Verification items for this drawing (mm, ordinates from the low corner). A direction names the side the tool comes from. Round coordinates to 2 decimals unless told otherwise and drop trailing zeros. Order: outer loops, then holes, each group sorted by start corner. A loop starts at its lowest first (then second) coordinate and runs counter-clockwise, first axis right, second up. Notation, with made-up numbers: (-13.75, 55) - (9.25, 55) arc R10 ccw to (9.25, 62) - close; hole circle Ø8 at (73.25, 43). An arc over 180 degrees is marked (long way). Return JSON: item names as keys, results as strings. Group by question number.
Q1. Sectioned sample at B-B, the plane y = 9. Record the cut outline in (x, z), then the cut area to 3 significant figures.
Q2. Sectioned sample at D-D, the plane x = 6. Record the cut outline in (y, z).
Q3. Draft check along X on the marked faces 4, 5 and 6. Enter one of: pulls with the +X half, pulls with the -X half, needs draft (parallel to the pull), parting line crosses it, or undercut.
Q4. Tool access check on the marked faces 1, 2 and 3. Record the directions out of +Z, -Z, +X, -X, +Y, -Y that give a thin tool (end or side, any length) a straight path to the whole face; none if there is none.
Q5. Gauge pin test, flat ends, axial feed: pin 1 Ø8 at (y, z) = (7.5, 35) entering from +X; pin 2 Ø3 at (x, y) = (58, 18) entering from -Z; pin 3 Ø1.5 at (x, z) = (1.5, 42.5) entering from -Y. Record the tip position at first contact, or that the pin passes through.
Q6. Sectioned sample at A-A, the plane z = 58.75. Record the cut outline in (x, y).
Q7. Material ranges on line 1 along Z through (x, y) = (5, 20); line 2 along X through (y, z) = (1.5, 66.5); line 3 along X through (y, z) = (15.5, 69.5), recorded low to high.
Q8. Sectioned sample at C-C, the plane y = 18.75. Record the cut outline in (x, z).
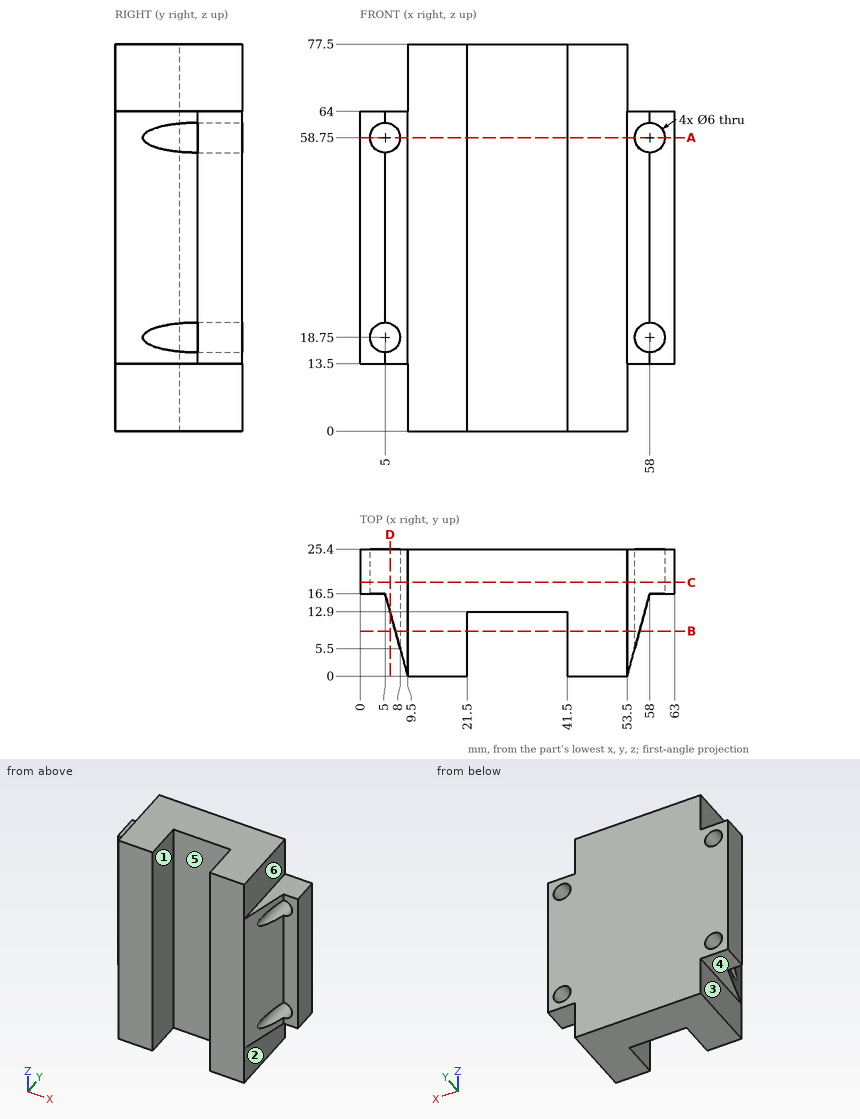
Reply:
{
 "1": {"outline": "(7.05, 13.5) - (9.5, 13.5) - (9.5, 0) - (21.5, 0) - (21.5, 77.5) - (9.5, 77.5) - (9.5, 64) - (7.05, 64) - (7.05, 60.94) arc R3 cw to (7.05, 56.56) - (7.05, 20.94) arc R3 cw to (7.05, 16.56) - close; (41.5, 0) - (53.5, 0) - (53.5, 13.5) - (55.95, 13.5) - (55.95, 16.56) arc R3 cw to (55.95, 20.94) - (55.95, 56.56) arc R3 cw to (55.95, 60.94) - (55.95, 64) - (53.5, 64) - (53.5, 77.5) - (41.5, 77.5) - close", "area": "2,100 mm^2"},
 "2": {"outline": "(12.83, 13.5) - (25.4, 13.5) - (25.4, 15.92) - (12.83, 15.92) - close; (12.83, 21.58) - (25.4, 21.58) - (25.4, 55.92) - (12.83, 55.92) - close; (12.83, 61.58) - (25.4, 61.58) - (25.4, 64) - (12.83, 64) - close"},
 "3": {"face 4": "needs draft", "face 5": "undercut", "face 6": "pulls with the +X half"},
 "4": {"face 1": "+Z, -Z, -Y", "face 2": "-Z, +X, +Y, -Y", "face 3": "-Z, -X, +Y, -Y"},
 "5": {"pin 1": "x = 56.64", "pin 2": "z = 13.5", "pin 3": "y = 16.5"},
 "6": {"outline": "(0, 16.5) - (2, 16.5) - (2, 25.4) - (0, 25.4) - close; (8, 5.5) - (9.5, 0) - (21.5, 0) - (21.5, 12.9) - (41.5, 12.9) - (41.5, 0) - (53.5, 0) - (55, 5.5) - (55, 25.4) - (8, 25.4) - close; (61, 16.5) - (63, 16.5) - (63, 25.4) - (61, 25.4) - close"},
 "7": {"line 1": "13.5 to 15.75, 21.75 to 55.75, 61.75 to 64", "line 2": "9.5 to 21.5, 41.5 to 53.5", "line 3": "9.5 to 53.5"},
 "8": {"outline": "(0, 13.5) - (9.5, 13.5) - (9.5, 0) - (53.5, 0) - (53.5, 13.5) - (63, 13.5) - (63, 64) - (53.5, 64) - (53.5, 77.5) - (9.5, 77.5) - (9.5, 64) - (0, 64) - close; hole circle Ø6 at (5, 18.75); hole circle Ø6 at (5, 58.75); hole circle Ø6 at (58, 18.75); hole circle Ø6 at (58, 58.75)"}
}
